For this review, take the finished solid that the model builds, in its own axes (mm). A direction names the side the tool comes from. Coordinates: 2 decimals unless noted, no trailing zeros. Loops run counter-clockwise (first coordinate to the right, second up) from the corner with the lowest first, then second, coordinate; pieces in that order, holes last. Notation, with made-up numbers: M 13,53 L 44,53 A33 cw 44,88 Z; hole C -16.5,60 d6. An arc over 180 degrees is marked long. Put each result on its own line as item: value.
Autodesk Inventor part; units mm, degrees
ref_plane "YZ Plane" through (0, 0, 0) normal (1, 0, 0) x (0, 1, 0)
ref_plane "XZ Plane" through (0, 0, 0) normal (0, 1, 0) x (-1, 0, 0)
ref_plane "XY Plane" through (0, 0, 0) normal (0, 0, 1) x (1, 0, 0)
sketch "Sketch1" plane through (0, 0, 0) normal (1, 0, 0) x (0, 1, 0)
  circle A0 centre (0, 0) radius 3.85 construction
  line L0 (-3.85, 0) -> (-1.925, 3.3342)
  line L1 (-1.925, 3.3342) -> (1.925, 3.3342)
  line L2 (1.925, 3.3342) -> (3.85, 0)
  line L3 (3.85, 0) -> (1.925, -3.3342)
  line L4 (1.925, -3.3342) -> (-1.925, -3.3342)
  line L5 (-1.925, -3.3342) -> (-3.85, 0)
  circle A1 centre (0, 0) radius 2
  dimension "d0" = 7.7
  dimension "d1" = 4
extrude "Extrusion1" add sketch "Sketch1" along normal mid plane 3
sketch "Sketch2" plane through (1.5, 0, 0) normal (1, 0, 0) x (0, 0, -1)
  circle A0 centre (0, 0) radius 3.3342
  circle A1 centre (0, 0) radius 2
extrude "Extrusion2" add sketch "Sketch2" along normal blind 1.3
fillet "Fillet1" radius 0.2 1 edges at (2.8, 0, 3.3342)
thread "Thread1"
properties part number "Nut 4mm self locking"
(1) Tool access review of faces 4 (the flat face through (1.5, 3.5, 0)), 5 (the flat face through (1.5, 1.8, -3)), 6 (the cylindrical face through (2.04, 1.28, -3.08)), 7 (the flat face through (1.5, -1.8, -3)), 8 (the flat face through (1.5, -1.8, 3)): name each direction out of +Z, -Z, +X, -X, +Y, -Y from which nothing blocks a thin tool from reaching the whole face with its end or side.
Determined:
face 4: +X, +Y
face 5: -Z, +X, +Y
face 6: +X
face 7: -Z, +X, -Y
face 8: +Z, +X, -Y
(2) Add section A-A (x = -1.2). Write out the cut boundary in (y, z) (3 decimals).
Determined:
outline: M -3.85,0 L -1.925,-3.334 L 1.925,-3.334 L 3.85,0 L 1.925,3.334 L -1.925,3.334 Z; hole C 0,0 d4
(3) Draft analysis for pull direction Z (two halves, no side actions). For faces 1 (the cylindrical face through (0.62, 0.944, -1.763)), 2 (the flat face through (-0.021, 2.901, -1.644)), 3 (the flat face through (1.5, 1.8, 3)), state which applies: +Z half, -Z half, draft (parallel to the pull), parting line (faces both ways), or undercut.
Determined:
face 1: undercut
face 2: -Z half
face 3: draft
(4) For pin 1 (2 mm diameter, centred on x = -0.5, z = -2, fed in from +Y); pin 2 (1 mm diameter, centred on x = 0, z = -2.5, fed in from -Y); pin 3 (1.5 mm diameter, centred on x = 0, z = -1, fed in from +Y), all flat-tipped, find the tip position at first contact; note any pin that passes through.
Determined:
pin 1: stops at y = 3.27
pin 2: stops at y = -2.7
pin 3: stops at y = 3.71
(5) Wall thickness on line 1 along Z through (x, y) = (0.7, 0); line 2 along Y through (x, z) = (1.85, -1.75); line 3 along Z through (x, y) = (-0.55, 0.5): over which ranges is each line inside the solid? List them lowest first. Write a range as [from, to].
Determined:
line 1: z = [-3.33, -2], [2, 3.33]
line 2: y = [-2.84, -0.97], [0.97, 2.84]
line 3: z = [-3.33, -1.94], [1.94, 3.33]
